Geometry check sheet. Reference: the model listing, model coordinates, mm. A direction names the side the tool comes from. Give positions to 0.01 mm unless a question says otherwise; leave off trailing zeros. Write each loop counter-clockwise with the first axis right and the second up, starting at its lowest first coordinate (ties: lowest second). Pieces come first, ordered by that corner, then holes. Notation, with made-up numbers: M 12,-31.75 L 27,-31.75 A23 cw 27,-2.75 Z; hole C -10.75,50 d2. An arc over 180 degrees is marked long. Use one line per item in the form item = value. Start each with the question number.
```python
from build123d import *

# Parameters (mm, degrees)
CROQUIS1_W              = 8
CROQUIS1_H              = 75
SALIENTE_EXTRUIR1_DEPTH = 3
CROQUIS2_R              = 2
CORTAR_EXTRUIR1_DEPTH   = 43.793106922
CROQUIS3_W              = 8
CROQUIS3_H              = 2
SALIENTE_EXTRUIR2_DEPTH = 1
CROQUIS4_W              = 8
CROQUIS4_H              = 3
SALIENTE_EXTRUIR3_DEPTH = 2.5
CROQUIS5_W              = 8
CROQUIS5_H              = 2
SALIENTE_EXTRUIR4_DEPTH = 10
CROQUIS7_R              = 2
CORTAR_EXTRUIR3_DEPTH   = 18.5
REDONDEO2_R             = 4
REDONDEO5_R             = 4


with BuildPart() as part:
    # Croquis1 → Saliente-Extruir1 (new body)
    with BuildSketch(Plane.XY):
        with Locations((0, -5)):
            Rectangle(CROQUIS1_W, CROQUIS1_H)
    extrude(amount=SALIENTE_EXTRUIR1_DEPTH)

    # Croquis2 → Cortar-Extruir1 (cut, through all)
    with BuildSketch(Plane.XY.offset(3)):
        with Locations((0, -38.5)):
            Circle(CROQUIS2_R)
    extrude(amount=-CORTAR_EXTRUIR1_DEPTH, mode=Mode.SUBTRACT)

    # Croquis3 → Saliente-Extruir2 (add)
    with BuildSketch(Plane.XY.offset(3)):
        with Locations((0, 6)):
            Rectangle(CROQUIS3_W, CROQUIS3_H)
    saliente_extruir2 = extrude(amount=SALIENTE_EXTRUIR2_DEPTH)

    # Simetría1: Saliente-Extruir2 across plane
    add(saliente_extruir2.mirror(Plane.XY.offset(1.5)))

    # Croquis4 → Saliente-Extruir3 (add)
    with BuildSketch(Plane(origin=(0, 0, 0), x_dir=(-1, 0, 0), z_dir=(0, 0, -1))):
        with Locations((0, 31)):
            Rectangle(CROQUIS4_W, CROQUIS4_H)
    saliente_extruir3 = extrude(amount=SALIENTE_EXTRUIR3_DEPTH)

    # Croquis5 → Saliente-Extruir4 (add)
    with BuildSketch(Plane(origin=(0, 32.5, 0), x_dir=(1, 0, 0), z_dir=(0, 1, 0))):
        with Locations((0, 1.5)):
            Rectangle(CROQUIS5_W, CROQUIS5_H)
    saliente_extruir4 = extrude(amount=SALIENTE_EXTRUIR4_DEPTH)

    # Croquis7 → Cortar-Extruir3 (cut)
    with BuildSketch(Plane(origin=(0, 0, -2.5), x_dir=(-1, 0, 0), z_dir=(0, 0, -1))):
        with Locations((0, 38.5)):
            Circle(CROQUIS7_R)
    cortar_extruir3 = extrude(amount=-CORTAR_EXTRUIR3_DEPTH, mode=Mode.SUBTRACT)

    # Redondeo2
    redondeo2_edges = [part.edges().sort_by_distance(p)[0] for p in [
        (4, 42.5, -1.5),
        (-4, 42.5, -1.5),
        (-4, -42.5, 1.5),
        (4, -42.5, 1.5),
    ]]
    fillet(redondeo2_edges, radius=REDONDEO2_R - 0.0001)  # a hair under: the kernel refuses the full size

    # Simetría3: Saliente-Extruir3, Saliente-Extruir4, Cortar-Extruir3 across plane
    add(saliente_extruir3.mirror(Plane.XY.offset(1.5)))
    add(saliente_extruir4.mirror(Plane.XY.offset(1.5)))
    add(cortar_extruir3.mirror(Plane.XY.offset(1.5)), mode=Mode.SUBTRACT)

    # Redondeo5
    redondeo5_edges = [part.edges().sort_by_distance(p)[0] for p in [
        (-4, 42.5, 4.5),
        (4, 42.5, 4.5),
    ]]
    fillet(redondeo5_edges, radius=REDONDEO5_R - 0.0001)  # a hair under: the kernel refuses the full size


solid = part.part
```
(1) Sectioned sample at B-B, the plane x = 1. State how many separate pieces and enclosed holes the cut face has, plus the area to 3 significant figures.
(2) Sectioned sample at C-C, the plane y = 15. Record the boundary of the cut face in (x, z), plus the area to 3 significant figures.
(3) Tool access check on faces 1 (the flat face through (0, 36, 3.5)), 2 (the flat face through (0, -18, 0)), 3 (the flat face through (0, -18, 3)). Record the directions out of +Z, -Z, +X, -X, +Y, -Y that give a thin tool (end or side, any length) a straight path to the whole face; none if there is none.
(4) Draft check along X on faces 4 (the cylindrical face through (0.434, 36.548, 4.514)), 5 (the flat face through (0, 6, -1)), 6 (the cylindrical face through (-2.859, -41.297, 1.521)). Enter one of: released by +X, released by -X, zero draft, split by the parting line, or undercut.
(5) Depth check by flat-ended pin: pin 1 (2 mm diameter, centred on x = -1.5, y = -7, fed in from +Z); pin 2 (2 mm diameter, centred on x = 0, y = -31.5, fed in from -Z); pin 3 (1 mm diameter, centred on x = 1, y = 6.5, fed in from -Z); pin 4 (3 mm diameter, centred on x = 0, y = -38.5, fed in from +Z). Enter the tip coordinate at first touch or a pass-through.
(6) Thickness scan on probe 1 along X at (y, z) = (38.5, 4.35); probe 2 along Y at (x, z) = (0, 5.1); probe 3 along Y at (x, z) = (-1.75, -0.25). Record the ranges inside material, lowest first. Write a range as [from, to].
Numbers:
q1.separate_pieces = 4
q1.enclosed_holes = 0
q1.area = 259 mm2
q2.outline = M -4,0 L 4,0 L 4,3 L -4,3 Z
q2.area = 24.0 mm2
q3.face_1 = +X, -X, +Y
q3.face_2 = -Z, +X, -X, -Y
q3.face_3 = +Z, +X, -X, -Y
q4.face_4 = undercut
q4.face_5 = zero draft
q4.face_6 = released by -X
q5.pin_1 = 3
q5.pin_2 = 0
q5.pin_3 = -1
q5.pin_4 = through
q6.probe_1 = [-4, -2], [2, 4]
q6.probe_2 = [29.5, 36.5], [40.5, 42.5]
q6.probe_3 = [5, 7], [29.5, 32.5]
